Design review of the part built by this model. Coordinates are the model's own, in mm. A direction names the side the tool comes from. Coordinates: 2 decimals unless noted, no trailing zeros. Loops run counter-clockwise (first coordinate to the right, second up) from the corner with the lowest first, then second, coordinate; pieces in that order, holes last. Notation, with made-up numbers: M 47.5,-3.5 L 63.5,-3.5 A16 cw 63.5,16.5 Z; hole C -2.75,63 d11. An arc over 180 degrees is marked long. One line per item, written item: value.
```python
from build123d import *

# Parameters (mm, degrees)
BOSS_EXTRUDE1_DEPTH = 16


with BuildPart() as part:
    # Sketch1 → Boss-Extrude1 (new body)
    with BuildSketch(Plane.XY):
        with BuildLine():
            Line((-2.05, 2.836811591), (-2.05, 2.05))
            Line((-2.05, 2.05), (-2.836811591, 2.05))
            ThreePointArc((-2.836811591, 2.05), (-3.5, 0), (-2.836811591, -2.05))
            Line((-2.836811591, -2.05), (-2.05, -2.05))
            Line((-2.05, -2.05), (-2.05, -2.836811591))
            ThreePointArc((-2.05, -2.836811591), (0, -3.5), (2.05, -2.836811591))
            Line((2.05, -2.836811591), (2.05, -2.05))
            Line((2.05, -2.05), (2.836811591, -2.05))
            ThreePointArc((2.836811591, -2.05), (3.5, 0), (2.836811591, 2.05))
            Line((2.836811591, 2.05), (2.05, 2.05))
            Line((2.05, 2.05), (2.05, 2.836811591))
            ThreePointArc((2.05, 2.836811591), (0, 3.5), (-2.05, 2.836811591))
        make_face()
        with BuildLine():
            Line((-0.9, 2.170829335), (-0.9, 0.9))
            Line((-0.9, 0.9), (-2.170829335, 0.9))
            ThreePointArc((-2.170829335, 0.9), (-2.35, 0), (-2.170829335, -0.9))
            Line((-2.170829335, -0.9), (-0.9, -0.9))
            Line((-0.9, -0.9), (-0.9, -2.170829335))
            ThreePointArc((-0.9, -2.170829335), (0, -2.35), (0.9, -2.170829335))
            Line((0.9, -2.170829335), (0.9, -0.9))
            Line((0.9, -0.9), (2.170829335, -0.9))
            ThreePointArc((2.170829335, -0.9), (2.35, 0), (2.170829335, 0.9))
            Line((2.170829335, 0.9), (0.9, 0.9))
            Line((0.9, 0.9), (0.9, 2.170829335))
            ThreePointArc((0.9, 2.170829335), (0, 2.35), (-0.9, 2.170829335))
        make_face(mode=Mode.SUBTRACT)
    extrude(amount=BOSS_EXTRUDE1_DEPTH)


solid = part.part
```
(1) We need section D-D on x = -3. State the section outline as (y, z) points.
Reply:
outline: M -1.8,0 L 1.8,0 L 1.8,16 L -1.8,16 Z
(2) Insertion check: pin 1 (0.6 mm diameter, centred on x = -2, z = 12, fed in from -Y); pin 2 (1.5 mm diameter, centred on x = 2.5, z = 4.5, fed in from -Y); pin 3 (1.4 mm diameter, centred on y = -1.5, z = 6, fed in from +X). Each pin has a flat end and moves straight along its axis. Give the tip position at first contact, or say it passes through.
Reply:
pin 1: stops at y = -3.06
pin 2: stops at y = -3.03
pin 3: stops at x = 3.41
(3) We need section A-A on z = 14. State the section outline as (x, y) points, then the cut area to 3 significant figures.
Reply:
outline: M -2.84,-2.05 L -2.05,-2.05 L -2.05,-2.84 A3.5 ccw 2.05,-2.84 L 2.05,-2.05 L 2.84,-2.05 A3.5 ccw 2.84,2.05 L 2.05,2.05 L 2.05,2.84 A3.5 ccw -2.05,2.84 L -2.05,2.05 L -2.84,2.05 A3.5 ccw Z; hole M -2.17,-0.9 L -0.9,-0.9 L -0.9,-2.17 A2.35 ccw 0.9,-2.17 L 0.9,-0.9 L 2.17,-0.9 A2.35 ccw 2.17,0.9 L 0.9,0.9 L 0.9,2.17 A2.35 ccw -0.9,2.17 L -0.9,0.9 L -2.17,0.9 A2.35 ccw Z
area: 23.9 mm2
(4) To check wall thickness, follow line 1 along X through (y, z) = (-2.75, 14.25); line 2 along Y through (x, z) = (1.25, 7.25); line 3 along Y through (x, z) = (-0.25, 6.5). State the ranges of each line that lie inside material, in increasing order. Write a range as [from, to].
Reply:
line 1: x = [-2.05, 2.05]
line 2: y = [-3.27, -0.9], [0.9, 3.27]
line 3: y = [-3.49, -2.34], [2.34, 3.49]
(5) Mouldability with a two-part tool opening along X and no side actions: class faces 1 (the cylindrical face through (0, -3.5, 7.9)), 2 (the flat face through (1.5, -1.5, 0)), 3 (the flat face through (-2, 0.9, 8)) as released by +X, released by -X, zero draft, split by the parting line, or undercut.
Reply:
face 1: split by the parting line
face 2: zero draft
face 3: undercut
(6) Tool access review of faces 4 (the flat face through (0.9, 2, 8)), 5 (the cylindrical face through (-3.5, 0, 7.9)): name each direction out of +Z, -Z, +X, -X, +Y, -Y from which nothing blocks a thin tool from reaching the whole face with its end or side.
Reply:
face 4: +Z, -Z
face 5: +Z, -Z, -X
(7) We need section B-B on x = 0. State the section outline as (y, z) points, then the cut area to 3 significant figures.
Reply:
outline: M -3.5,0 L -2.35,0 L -2.35,16 L -3.5,16 Z; M 2.35,0 L 3.5,0 L 3.5,16 L 2.35,16 Z
area: 36.8 mm2
